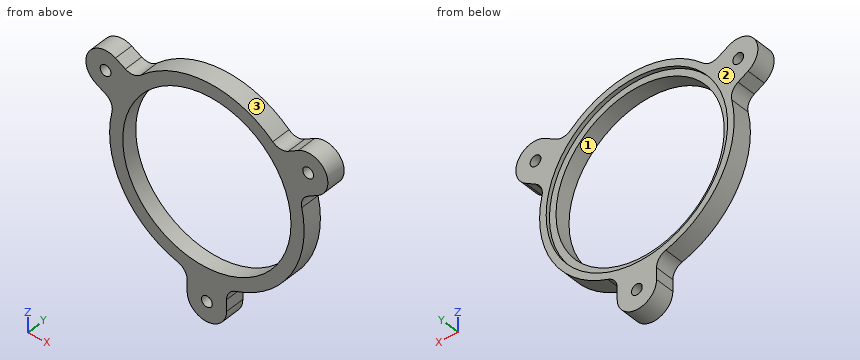
```python
from build123d import *

# Parameters (mm, degrees)
SKETCH1_R           = 69
SKETCH1_R_2         = 4.1
BOSS_EXTRUDE1_DEPTH = 15
SKETCH2_R           = 69
SKETCH2_R_2         = 64
BOSS_EXTRUDE5_DEPTH = 12


with BuildPart() as part:
    # Sketch1 → Boss-Extrude1 (new body)
    with BuildSketch(Plane(origin=(0, 0, 0), x_dir=(1, 0, 0), z_dir=(0, 1, 0))):
        with BuildLine():
            Line((84.576260937, -31.509618943), (76.949622029, -27.106376917))
            ThreePointArc((76.949622029, -27.106376917), (72.790004977, -22.458779787), (72.193714645, -16.25015587))
            ThreePointArc((72.193714645, -16.25015587), (64.08587988, 37), (22.023809524, 70.646668811))
            ThreePointArc((22.023809524, 70.646668811), (16.945128655, 74.267383345), (15, 80.193515947))
            Line((15, 80.193515947), (15, 89))
            ThreePointArc((15, 89), (0, 104), (-15, 89))
            Line((-15, 89), (-15, 80.193515947))
            ThreePointArc((-15, 80.193515947), (-16.945128655, 74.267383345), (-22.023809524, 70.646668811))
            ThreePointArc((-22.023809524, 70.646668811), (-64.071073413, 37.025633711), (-72.206692839, -16.192390475))
            ThreePointArc((-72.206692839, -16.192390475), (-72.806342922, -22.396872115), (-76.964354033, -27.040805388))
            Line((-76.964354033, -27.040805388), (-84.608337243, -31.454061152))
            Line((-84.608337243, -31.454061152), (-84.576260937, -31.509618943))
            ThreePointArc((-84.576260937, -31.509618943), (-90.066641994, -52), (-69.576260937, -57.490381057))
            Line((-69.576260937, -57.490381057), (-61.949622029, -53.08713903))
            ThreePointArc((-61.949622029, -53.08713903), (-55.844876322, -51.808603558), (-50.169905121, -54.396512941))
            ThreePointArc((-50.169905121, -54.396512941), (0, -74), (50.169905121, -54.396512941))
            ThreePointArc((50.169905121, -54.396512941), (55.844876322, -51.808603558), (61.949622029, -53.08713903))
            Line((61.949622029, -53.08713903), (69.576260937, -57.490381057))
            ThreePointArc((69.576260937, -57.490381057), (90.066641994, -52), (84.576260937, -31.509618943))
        make_face()
        Circle(SKETCH1_R, mode=Mode.SUBTRACT)
        with Locations((-77.076260937, -44.5)):
            Circle(SKETCH1_R_2, mode=Mode.SUBTRACT)
        with Locations((77.076260937, -44.5)):
            Circle(SKETCH1_R_2, mode=Mode.SUBTRACT)
        with Locations((0, 89)):
            Circle(SKETCH1_R_2, mode=Mode.SUBTRACT)
    extrude(amount=BOSS_EXTRUDE1_DEPTH)

    # Sketch2 → Boss-Extrude5 (add)
    with BuildSketch(Plane(origin=(0, 0, 0), x_dir=(1, 0, 0), z_dir=(0, 1, 0))):
        Circle(SKETCH2_R)
        Circle(SKETCH2_R_2, mode=Mode.SUBTRACT)
    extrude(amount=BOSS_EXTRUDE5_DEPTH)


solid = part.part
```
Could you check a few things on this model? Use its own coordinates, in mm. Face numbers are marked on the shaded views. Coordinates: 2 decimals unless noted, no trailing zeros. Write each loop counter-clockwise with the first axis right and the second up, starting at its lowest first coordinate (ties: lowest second). Pieces come first, ordered by that corner, then holes. Notation, with made-up numbers: (55, -11.5) - (108, -11.5) arc R27 cw to (108, 18.5) - close; hole circle Ø10 at (5.25, -9.5). An arc over 180 degrees is marked (long way). Use a Markdown table: item, result.
Q1. Imagine slicing it at B-B (x = -2). List the corners of the cut face in (y, z) for me, and give its area (3 significant figures).
Geometry check:
| item | result |
|---|---|
| outline | (0, -103.87) - (15, -103.87) - (15, -92.58) - (0, -92.58) - close; (0, -85.42) - (15, -85.42) - (15, -68.97) - (12, -68.97) - (12, -63.97) - (0, -63.97) - close; (0, 63.97) - (12, 63.97) - (12, 68.97) - (15, 68.97) - (15, 73.97) - (0, 73.97) - close |
| area | 611 mm2 |
Q2. Please list where these lines run through material, in increasing order: L1, parallel to Z at x = -0.5, y = 2.25; L2, parallel to X at y = 6.25, z = 0; L3, parallel to X at y = 13.3, z = 0.
Geometry check:
| item | result |
|---|---|
| L1 | z = -103.99 to -93.07, -84.93 to -64, 64 to 74 |
| L2 | x = -74 to -64, 64 to 74 |
| L3 | x = -74 to -69, 69 to 74 |
Q3. Thinking about a two-plate mould opening in Z: for the marked faces 1, 2 and 3, which applies, +Z half, -Z half, draft (parallel to the pull), parting line (faces both ways), or undercut?
Geometry check:
| item | result |
|---|---|
| face 1 | undercut |
| face 2 | draft |
| face 3 | +Z half |
Q4. Imagine slicing it at D-D (y = 6.25). List the corners of the cut face in (x, z) for me.
Geometry check:
| item | result |
|---|---|
| outline | (-84.61, 31.45) - (-76.96, 27.04) arc R10 cw to (-72.21, 16.19) arc R74 ccw to (-22.02, -70.65) arc R10 cw to (-15, -80.19) - (-15, -89) arc R15 ccw to (15, -89) - (15, -80.19) arc R10 cw to (22.02, -70.65) arc R74 ccw to (72.19, 16.25) arc R10 cw to (76.95, 27.11) - (84.58, 31.51) arc R15 ccw to (69.58, 57.49) - (61.95, 53.09) arc R10 cw to (50.17, 54.4) arc R74 ccw to (-50.17, 54.4) arc R10 cw to (-61.95, 53.09) - (-69.58, 57.49) arc R15 ccw to (-84.58, 31.51) - close; hole circle Ø8.2 at (-77.08, 44.5); hole circle Ø128 at (0, 0); hole circle Ø8.2 at (0, -89); hole circle Ø8.2 at (77.08, 44.5) |
Q5. Imagine slicing it at C-C (z = 44.5). List the corners of the cut face in (x, y) for me, and give its area (3 significant figures).
Geometry check:
| item | result |
|---|---|
| outline | (-92.08, 0) - (-81.18, 0) - (-81.18, 15) - (-92.08, 15) - close; (-72.98, 0) - (-46, 0) - (-46, 12) - (-52.73, 12) - (-52.73, 15) - (-72.98, 15) - close; (46, 0) - (72.98, 0) - (72.98, 15) - (52.73, 15) - (52.73, 12) - (46, 12) - close; (81.18, 0) - (92.08, 0) - (92.08, 15) - (81.18, 15) - close |
| area | 1,100 mm2 |
Q6. I'm going to push flat-ended pins straight in: pin 1 Ø1.5 at (y, z) = (7, 4) entering from +X; pin 2 Ø5 at (x, y) = (-23, 11.5) entering from -Z; pin 3 Ø9.5 at (x, z) = (-77.08, 44.5) entering from -Y; pin 4 Ø1 at (x, y) = (56.5, 12.5) entering from +Z. Where does each tip first touch, or does it pass through?
Geometry check:
| item | result |
|---|---|
| pin 1 | stops at x = 73.93 |
| pin 2 | stops at z = -71.26 |
| pin 3 | stops at y = 0 |
| pin 4 | stops at z = 51.79 |
Q7. Imagine slicing it at A-A (z = 0). List the corners of the cut face in (x, y) for me.
Geometry check:
| item | result |
|---|---|
| outline | (-74, 0) - (-64, 0) - (-64, 12) - (-69, 12) - (-69, 15) - (-74, 15) - close; (64, 0) - (74, 0) - (74, 15) - (69, 15) - (69, 12) - (64, 12) - close |
